```python
from build123d import *

# Parameters (mm, degrees)
SKETCH1_W           = 110
SKETCH1_H           = 85
BOSS_EXTRUDE1_DEPTH = 45
SKETCH2_W           = 105
SKETCH2_H           = 80
CUT_EXTRUDE1_DEPTH  = 42.5
FILLET1_R           = 2.5
SKETCH3_R           = 3.75
BOSS_EXTRUDE3_DEPTH = 2.5
SKETCH5_R           = 2.5
CUT_EXTRUDE2_DEPTH  = 30
FILLET2_R           = 2.5
FILLET3_R           = 1
FILLET4_R           = 1
SKETCH12_R          = 6
CUT_EXTRUDE3_DEPTH  = 30
SKETCH13_R          = 3.35
CUT_EXTRUDE4_DEPTH  = 30


# Read off the part's stored shape, not the designer's step: Cut-Sweep1
# Some blends are built 0.0001 mm under size
with BuildPart() as part:
    # Sketch1 → Boss-Extrude1 (new body)
    with BuildSketch(Plane(origin=(0, 0, 0), x_dir=(1, 0, 0), z_dir=(0, 1, 0))):
        Rectangle(SKETCH1_W, SKETCH1_H)
    extrude(amount=BOSS_EXTRUDE1_DEPTH)

    # Sketch2 → Cut-Extrude1 (cut)
    with BuildSketch(Plane(origin=(0, 45, 0), x_dir=(1, 0, 0), z_dir=(0, 1, 0))):
        Rectangle(SKETCH2_W, SKETCH2_H)
    extrude(amount=-CUT_EXTRUDE1_DEPTH, mode=Mode.SUBTRACT)

    # Fillet1
    fillet1_edges = [part.edges().sort_by_distance(p)[0] for p in [
        (55, 45, 0),
        (0, 0, 42.5),
        (-55, 0, 0),
        (0, 0, -42.5),
        (55, 0, 0),
        (55, 22.5, 42.5),
        (-55, 22.5, 42.5),
        (-55, 22.5, -42.5),
        (55, 22.5, -42.5),
    ]]
    fillet(fillet1_edges, radius=FILLET1_R - 0.0001)  # a hair under: the kernel refuses the full size

    # Sketch3 → Boss-Extrude3 (add)
    with BuildSketch(Plane.ZY.offset(55)):
        with Locations(Location((0, 23.219153855, 0), (0, 0, 180))):
            Circle(SKETCH3_R)
    extrude(amount=BOSS_EXTRUDE3_DEPTH)

    # Sketch5 → Cut-Extrude2 (cut)
    with BuildSketch(Plane.ZY.offset(57.5)):
        with Locations((0, 23.219153855)):
            Circle(SKETCH5_R)
    extrude(amount=-CUT_EXTRUDE2_DEPTH, mode=Mode.SUBTRACT)

    # Cut-Sweep1 outline → Cut-Sweep1 (revolve, cut)
    with BuildSketch(Plane(origin=(0, 23.219153855, 0), x_dir=(0, 1, 0), z_dir=(0, 0, -1))):
        with BuildLine():
            ThreePointArc((3.75, -56.25), (2.866116524, -56.616116524), (2.5, -57.5))
            Line((2.5, -57.5), (3.75, -57.5))
            Line((3.75, -57.5), (3.75, -56.25))
        make_face()
    revolve(axis=Axis((0, 23.219153855, 0), (1, 0, 0)), mode=Mode.SUBTRACT)

    # Fillet2
    # the kernel refuses this fillet: 2.5 mm, written as the material it adds along each edge
    with BuildSketch(Plane(origin=(-55, 23.219153855, 0), x_dir=(0, 0, -1), z_dir=(0, 1, 0))) as fillet2_piece_1:
        with BuildLine():
            CenterArc((5.915063509, 2.5), FILLET2_R, 210, 60)
            Line((3.75, 1.25), (3.70669873, 1.225))
            ThreePointArc((3.70669873, 1.225), (3.7, 0.625), (3.7, 0))
            Line((3.7, 0), (3.75, -0.05))
            Line((3.75, -0.05), (5.915063509, -0.05))
            Line((5.915063509, -0.05), (5.915063509, 0))
        make_face()
    revolve(axis=Axis((-55, 23.219153855, 0), (-1, 0, 0)))

    # Fillet3
    fillet3_edges = [part.edges().sort_by_distance(p)[0] for p in [
        (-52.5, 23.219153855, -2.5),
    ]]
    fillet(fillet3_edges, radius=FILLET3_R)

    # Fillet4
    fillet4_edges = [part.edges().sort_by_distance(p)[0] for p in [
        (52.5, 23.75, -40),
        (52.5, 23.75, 40),
        (-52.5, 23.75, 40),
        (-52.5, 23.75, -40),
    ]]
    fillet(fillet4_edges, radius=FILLET4_R)

    # Sketch12 → Cut-Extrude3 (cut)
    with BuildSketch(Plane(origin=(55, 0, 0), x_dir=(0, 0, -1), z_dir=(1, 0, 0))):
        with Locations((20, 31.765581052)):
            Circle(SKETCH12_R)
    extrude(amount=-CUT_EXTRUDE3_DEPTH, mode=Mode.SUBTRACT)

    # Sketch13 → Cut-Extrude4 (cut)
    with BuildSketch(Plane.ZY.offset(55)):
        with Locations((-35, 23.964639065)):
            Circle(SKETCH13_R)
    extrude(amount=-CUT_EXTRUDE4_DEPTH, mode=Mode.SUBTRACT)


solid = part.part
```
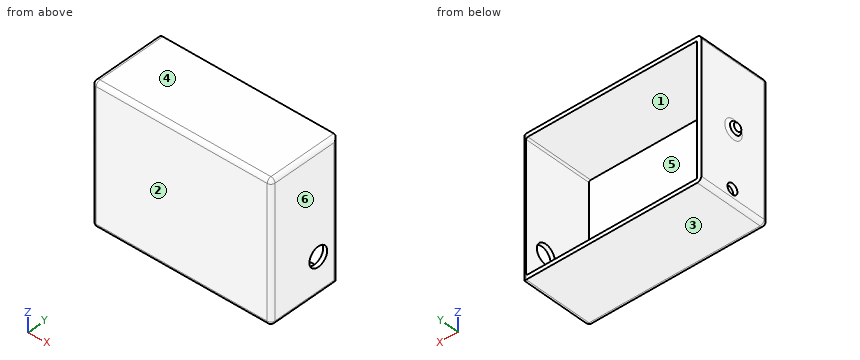
Geometry: final body of the model. Coordinates: model frame, mm. Face numbers are marked on the shaded views. A direction names the side the tool comes from. Coordinates: 2 decimals unless noted, no trailing zeros. Order: outer loops, then holes, each group sorted by start corner. A loop starts at its lowest first (then second) coordinate and runs counter-clockwise, first axis right, second up. Notation, with made-up numbers: (23, 70.25) - (74, 70.25) arc R17 ccw to (74, 81.25) - close; hole circle Ø3 at (77.25, 70). An arc over 180 degrees is marked (long way). Return JSON: item names as keys, results as strings. Group by question number.
1. Set-up query: the marked faces 1 and 2. Return all of +Z, -Z, +X, -X, +Y, -Y with unobstructed straight access to the full face (end or side cutting, diameter ignored); none if empty.
2. Cut plane D-D (x = -46). Output: boundary loops of the cut face in (y, z).
3. Pull-direction query (Z, two-part tool) for the marked faces 3, 4, 5 and 6; classes: pulls with the +Z half, pulls with the -Z half, needs draft (parallel to the pull), parting line crosses it, or undercut.
4. Pin query (flat end, axial travel): pin 1 (5 mm diameter, centred on y = 18, z = -5, fed in from -X); pin 2 (13 mm diameter, centred on y = 23, z = 8, fed in from -X); pin 3 (4 mm diameter, centred on y = 23.22, z = 0, fed in from -X); pin 4 (9.5 mm diameter, centred on y = 31.77, z = -20, fed in from +X). Return the tip coordinate at first contact, or that it passes through.
5. Cut plane B-B (y = 40). Output: boundary loops of the cut face in (x, z).
6. Material intervals for line 1 along Z through (x, y) = (33.5, 14.5); line 2 along X through (y, z) = (16, -16); line 3 along Y through (x, z) = (-54.25, -35), sorted ascending. Write a range as [from, to].
Resolved:
{
 "1": {"face 1": "+Y", "face 2": "+Z, -Z, +X, -X, -Y"},
 "2": {"outline": "(0, -40) arc R2.5 ccw to (2.5, -42.5) - (45, -42.5) - (45, -40) - (2.5, -40) - (2.5, 40) - (45, 40) - (45, 42.5) - (2.5, 42.5) arc R2.5 ccw to (0, 40) - close"},
 "3": {"face 3": "pulls with the -Z half", "face 4": "pulls with the +Z half", "face 5": "undercut", "face 6": "needs draft"},
 "4": {"pin 1": "stops at x = -55.3", "pin 2": "stops at x = -57.5", "pin 3": "stops at x = 52.5", "pin 4": "stops at x = -52.5"},
 "5": {"outline": "(-55, -40) arc R2.5 ccw to (-52.5, -42.5) - (52.5, -42.5) arc R2.5 ccw to (55, -40) - (55, 40) arc R2.5 ccw to (52.5, 42.5) - (-52.5, 42.5) arc R2.5 ccw to (-55, 40) - close; hole (-52.5, -39) arc R1 ccw to (-51.5, -40) - (51.5, -40) arc R1 ccw to (52.5, -39) - (52.5, 39) arc R1 ccw to (51.5, 40) - (-51.5, 40) arc R1 ccw to (-52.5, 39) - close"},
 "6": {"line 1": "z = [-42.5, -40], [40, 42.5]", "line 2": "x = [-55, -52.5], [52.5, 55]", "line 3": "y = [0.71, 20.61], [27.31, 45]"}
}
